Work out the finished part from the listing and answer in its coordinate system (mm). Round coordinates to 2 decimals unless told otherwise and drop trailing zeros. Order: outer loops, then holes, each group sorted by start corner. A loop starts at its lowest first (then second) coordinate and runs counter-clockwise, first axis right, second up. Notation, with made-up numbers: (74.5, 45) -> (95.5, 45) arc R21 cw to (95.5, 84) -> close; hole circle Ø3 at (0.5, -15). An arc over 180 degrees is marked (long way). Use a Markdown table: item, result. Add a question column.
Item 1: A cutting plane is placed at B-B, the plane x = -264.5. Determine the outline of the cut face in (y, z).
Item 2: A cutting plane is placed at A-A, the plane z = -9.5. Determine the outline of the cut face in (x, y).
Item 3: Flat-ended cylindrical pins translate along their axes: P1, Ø1.5, axis at x = 253, z = -1, coming from the +Y side; P2, Ø2.5, axis at y = 12.5, z = -4.5, coming from the +X side; P3, Ø4.5, axis at x = -382.25, y = 9, coming from the -Z side. Find the tip coordinate at first contact, or state that the pin passes through.
Item 4: Find the intervals of material crossed by L1, parallel to X at y = 9, z = 4.95; L2, parallel to Y at x = 382.25, z = 11.7; L3, parallel to Y at x = 382, z = 5, in increasing order. Write a range as [from, to].
from build123d import *

# Parameters (mm, degrees)
F1_DEPTH = 390
F2_W     = 31
F2_H     = 25
F3_DEPTH = 15.5
F4_W     = 31
F4_H     = 25
F5_DEPTH = 15.5
F6_R     = 2
F7_DEPTH = 10.001
F8_R     = 3.5
F9_DEPTH = 4
F10_R    = 1
F11_R    = 1


# Not quite as in the source:
# - a pattern or mirror of a feature is missing from the dataset's text; its kind, count and spacing are read off the source's solid


with BuildPart() as f1:
    # F0 (on Right) → F1 (new body, symmetric)
    with BuildSketch(Plane.YZ):
        Polygon((18.5, 12.5), (-18.5, 12.5), (-18.5, 2.5), (-15.5, 2.5), (-15.5, -22.5), (-10.5, -22.5), (-10.5, 2.5), (0, 2.5), (10.5, 2.5), (10.5, -22.5), (15.5, -22.5), (15.5, 2.5), (18.5, 2.5), align=None)
    extrude(amount=F1_DEPTH, both=True)

    # F2 (on face) → F3 (cut)
    with BuildSketch(Plane(origin=(-390, 0, 0), x_dir=(0, -1, 0), z_dir=(-1, 0, 0))):
        with Locations((0, -10)):
            Rectangle(F2_W, F2_H)
    extrude(amount=-F3_DEPTH, mode=Mode.SUBTRACT)

    # F4 (on face) → F5 (cut)
    with BuildSketch(Plane.YZ.offset(390)):
        with Locations((0, -10)):
            Rectangle(F4_W, F4_H)
    extrude(amount=-F5_DEPTH, mode=Mode.SUBTRACT)

    # F6 (on face) → F7 (cut, through all)
    with BuildSketch(Plane(origin=(0, 0, 2.5), x_dir=(1, 0, 0), z_dir=(0, 0, -1))):
        with Locations((-382.25, 9)):
            Circle(F6_R)
        with Locations((-382.25, -9)):
            Circle(F6_R)
    f7 = extrude(amount=-F7_DEPTH, mode=Mode.SUBTRACT)

    # F7_copies: F7 across plane
    add(f7.mirror(Plane(origin=(0, 0, 0), x_dir=(0, 0, 1), z_dir=(1, 0, 0))), mode=Mode.SUBTRACT)

    # F8 (on face) → F9 (cut)
    with BuildSketch(Plane.XY.offset(12.5)):
        with Locations((-382.25, -9)):
            Circle(F8_R)
        with Locations((-382.25, 9)):
            Circle(F8_R)
    f9 = extrude(amount=-F9_DEPTH, mode=Mode.SUBTRACT)

    # F9_copies: F9 across plane
    add(f9.mirror(Plane(origin=(0, 0, 0), x_dir=(0, 0, 1), z_dir=(1, 0, 0))), mode=Mode.SUBTRACT)

    # F10
    f10_edges = [f1.edges().sort_by_distance(p)[0] for p in [
        (390, 18.5, 7.5),
        (390, -18.5, 7.5),
        (374.5, 13, -22.5),
        (374.5, -13, -22.5),
        (-390, -18.5, 7.5),
        (-374.5, -13, -22.5),
        (-374.5, 13, -22.5),
        (-390, 18.5, 7.5),
    ]]
    fillet(f10_edges, radius=F10_R)

    # F11
    f11_edges = [f1.edges().sort_by_distance(p)[0] for p in [
        (-374.5, -10.5, -9.5),
        (-374.5, -15.5, -9.5),
        (-374.5, 15.5, -9.5),
        (-374.5, 10.5, -9.5),
        (-374.5, 13, -21.5),
        (-374.5, 13, 2.5),
        (-390, 0, 2.5),
        (-390, 0, 12.5),
        (0, -15.5, 2.5),
        (-389.707107, 18.207107, 12.5),
        (-389.707107, -18.207107, 12.5),
        (0, 18.5, 12.5),
        (0, -18.5, 12.5),
        (389.707107, 18.207107, 12.5),
        (389.707107, -18.207107, 12.5),
        (390, 0, 12.5),
        (-389.707107, 18.207107, 2.5),
        (-389.707107, -18.207107, 2.5),
        (0, 18.5, 2.5),
        (0, -18.5, 2.5),
        (389.707107, 18.207107, 2.5),
        (389.707107, -18.207107, 2.5),
        (390, 0, 2.5),
        (-374.5, -13, 2.5),
        (374.5, -13, 2.5),
        (0, -10.5, 2.5),
        (0, 10.5, 2.5),
        (374.5, 13, 2.5),
        (0, 15.5, 2.5),
        (374.5, -15.5, -9.5),
        (374.207107, -15.5, -22.207107),
        (0, -15.5, -22.5),
        (-374.207107, -15.5, -22.207107),
        (374.5, -10.5, -9.5),
        (0, -10.5, -22.5),
        (-374.207107, -10.5, -22.207107),
        (374.207107, -10.5, -22.207107),
        (374.5, 10.5, -9.5),
        (374.207107, 10.5, -22.207107),
        (0, 10.5, -22.5),
        (-374.207107, 10.5, -22.207107),
        (374.5, 15.5, -9.5),
        (0, 15.5, -22.5),
        (-374.207107, 15.5, -22.207107),
        (374.207107, 15.5, -22.207107),
    ]]
    fillet(f11_edges, radius=F11_R)


solid = f1.part
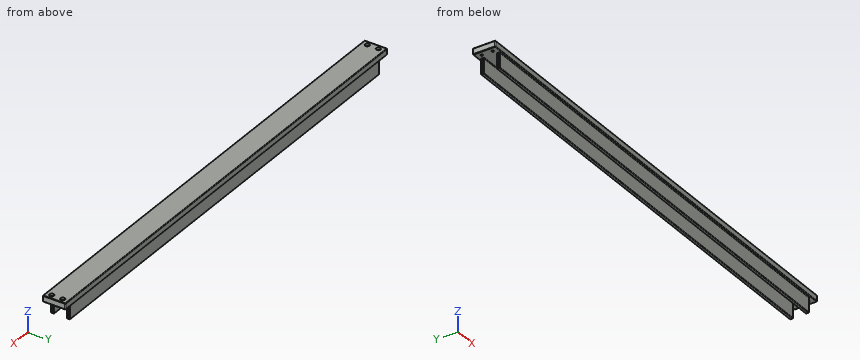
Reported:
| question | item | result |
|---|---|---|
| 1 | outline | (-18.5, 3.5) arc R1 ccw to (-17.5, 2.5) -> (-16.5, 2.5) arc R1 cw to (-15.5, 1.5) -> (-15.5, -21.5) arc R1 ccw to (-14.5, -22.5) -> (-11.5, -22.5) arc R1 ccw to (-10.5, -21.5) -> (-10.5, 1.5) arc R1 cw to (-9.5, 2.5) -> (9.5, 2.5) arc R1 cw to (10.5, 1.5) -> (10.5, -21.5) arc R1 ccw to (11.5, -22.5) -> (14.5, -22.5) arc R1 ccw to (15.5, -21.5) -> (15.5, 1.5) arc R1 cw to (16.5, 2.5) -> (17.5, 2.5) arc R1 ccw to (18.5, 3.5) -> (18.5, 11.5) arc R1 ccw to (17.5, 12.5) -> (-17.5, 12.5) arc R1 ccw to (-18.5, 11.5) -> close |
| 2 | outline | (-374.5, -14.5) arc R1 ccw to (-373.5, -15.5) -> (373.5, -15.5) arc R1 ccw to (374.5, -14.5) -> (374.5, -11.5) arc R1 ccw to (373.5, -10.5) -> (-373.5, -10.5) arc R1 ccw to (-374.5, -11.5) -> close; (-374.5, 11.5) arc R1 ccw to (-373.5, 10.5) -> (373.5, 10.5) arc R1 ccw to (374.5, 11.5) -> (374.5, 14.5) arc R1 ccw to (373.5, 15.5) -> (-373.5, 15.5) arc R1 ccw to (-374.5, 14.5) -> close |
| 3 | P1 | y = 15.5 |
| 3 | P2 | x = 374.5 |
| 3 | P3 | z = 2.5 |
| 4 | L1 | [-390, -384.25], [-380.25, 380.25], [384.25, 390] |
| 4 | L2 | [-18.48, -12.5], [-5.5, 5.5], [12.5, 18.48] |
| 4 | L3 | [-18.5, -10.98], [-7.02, 7.02], [10.98, 18.5] |
